Geometry check sheet. Reference: the model listing, model coordinates, mm. Face numbers are marked on the shaded views. A direction names the side the tool comes from. Coordinates: 2 decimals unless noted, no trailing zeros. Write each loop counter-clockwise with the first axis right and the second up, starting at its lowest first coordinate (ties: lowest second). Pieces come first, ordered by that corner, then holes. Notation, with made-up numbers: (-38, -5.5) -> (15, -5.5) arc R14 cw to (15, 1.5) -> close; hole circle Ø2 at (81.5, 74.25). An arc over 180 degrees is marked (long way). Put each result on its own line as item: value. Start each with the question number.
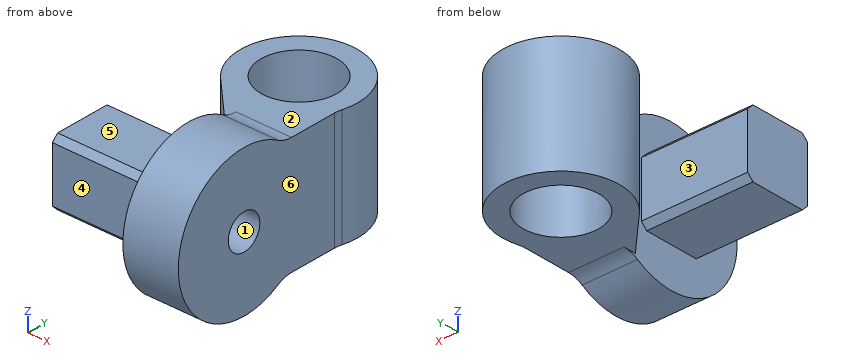
from build123d import *

# Parameters (mm, degrees)
SKETCH1_R           = 62.5
SKETCH1_R_2         = 15
BOSS_EXTRUDE1_DEPTH = 47.5
SKETCH2_R           = 32.5
BOSS_EXTRUDE2_DEPTH = 50
BOSS_EXTRUDE3_START = -47.5
BOSS_EXTRUDE3_DEPTH = 47.5
BOSS_EXTRUDE4_DEPTH = 100
FILLET1_R           = 25
SKETCH5_W           = 57
SKETCH5_H           = 57
BOSS_EXTRUDE5_DEPTH = 91
CHAMFER1_SIZE       = 5


with BuildPart() as part:
    # Sketch1 → Boss-Extrude1 (new body)
    with BuildSketch(Plane(origin=(0, 0, 0), x_dir=(0, 0, -1), z_dir=(1, 0, 0))):
        Circle(SKETCH1_R)
        Circle(SKETCH1_R_2, mode=Mode.SUBTRACT)
    extrude(amount=BOSS_EXTRUDE1_DEPTH)

    # Sketch2 → Boss-Extrude2 (add, symmetric)
    with BuildSketch(Plane.XY):
        with BuildLine():
            Line((-35.355339059, 69.644660941), (0, 34.289321881))
            Line((0, 34.289321881), (0, 55))
            ThreePointArc((0, 55), (19.134171618, 151.193976626), (-35.355339059, 69.644660941))
        make_face()
        with Locations((0, 105)):
            Circle(SKETCH2_R, mode=Mode.SUBTRACT)
    extrude(amount=BOSS_EXTRUDE2_DEPTH, both=True)

    # Sketch3 → Boss-Extrude3 (add)
    with BuildSketch(Plane(origin=(47.5, 0, 0), x_dir=(0, 0, -1), z_dir=(1, 0, 0)).offset(BOSS_EXTRUDE3_START)):
        with BuildLine():
            Line((-50, 55), (-50, 62.5))
            Line((-50, 62.5), (50, 62.5))
            Line((50, 62.5), (50, 55))
            Line((50, 55), (50, 37.5))
            ThreePointArc((50, 37.5), (40.792418173, 47.352176503), (29.685855218, 55))
            Line((29.685855218, 55), (-29.685855218, 55))
            ThreePointArc((-29.685855218, 55), (-40.792418173, 47.352176503), (-50, 37.5))
            Line((-50, 37.5), (-50, 55))
        make_face()
    extrude(amount=BOSS_EXTRUDE3_DEPTH)

    # Sketch4 → Boss-Extrude4 (add)
    with BuildSketch(Plane.XY.offset(50)):
        with BuildLine():
            Line((26.339134382, 62.5), (47.5, 62.5))
            Line((47.5, 62.5), (47.5, 89.387505004))
            ThreePointArc((47.5, 89.387505004), (39.291079432, 74.07733716), (26.339134382, 62.5))
        make_face()
    extrude(amount=-BOSS_EXTRUDE4_DEPTH)

    # Fillet1
    fillet1_edges = [part.edges().sort_by_distance(p)[0] for p in [
        (23.75, 37.5, 50),
        (23.75, 37.5, -50),
        (47.5, 89.387505004, 0),
    ]]
    fillet(fillet1_edges, radius=FILLET1_R)

    # Sketch5 → Boss-Extrude5 (add)
    with BuildSketch(Plane.ZY):
        Rectangle(SKETCH5_W, SKETCH5_H)
    extrude(amount=BOSS_EXTRUDE5_DEPTH)

    # Chamfer1
    chamfer1_edges = [part.edges().sort_by_distance(p)[0] for p in [
        (-45.5, -28.5, 28.5),
        (-45.5, 28.5, 28.5),
        (-45.5, 28.5, -28.5),
        (-45.5, -28.5, -28.5),
    ]]
    chamfer(chamfer1_edges, length=CHAMFER1_SIZE)


solid = part.part
Item 1: Go/stop test with flat-tipped pins: P1, Ø9, axis at y = -7, z = 6, coming from the +X side; P2, Ø23.5, axis at x = -38, y = -4.5, coming from the -Z side; P3, Ø6, axis at x = 35.5, z = -37, coming from the -Y side. Record where each tip stops, or that it passes through.
Item 2: Section check D-D, the plane z = 0. Enter the section's corners in (x, y), and give its area (3 significant figures).
Item 3: Mould release check, pull along Z, two halves, no side actions. Record for the marked faces 1, 2 and 3: released by +Z, released by -Z, zero draft, split by the parting line, or undercut.
Item 4: Section check C-C, the plane x = -53. Enter the section's corners in (y, z), and give its area (3 significant figures).
Item 5: Section check A-A, the plane x = 29. Enter the section's corners in (y, z).
Item 6: Access from +Z, -Z, +X, -X, +Y, -Y to the whole of each face (thin tool, end or side, straight path). Record for the marked faces 4, 5 and 6.
Item 7: Section check B-B, the plane y = 105. Enter the section's corners in (x, z).
Item 8: Scan lines: line 1 along Y through (x, z) = (0.5, -0.5); line 2 along Y through (x, z) = (26, 0); line 3 along Y through (x, z) = (-53.5, -4.5). Record each from-to range of solid material in increasing order. Write a range as [from, to].
From the geometry:
1. P1: x = 0
1. P2: z = -28.5
1. P3: y = -52.44
2. outline: (-91, -28.5) -> (0, -28.5) -> (0, -62.5) -> (47.5, -62.5) -> (47.5, -15) -> (0, -15) -> (0, 15) -> (47.5, 15) -> (47.5, 85.8) arc R25 cw to (48.33, 92.2) arc R50 ccw (long way) to (-35.36, 69.64) -> (0, 34.29) -> (0, 28.5) -> (-91, 28.5) -> close; hole circle Ø65 at (0, 105)
2. area: 14,600 mm²
3. face 1: undercut
3. face 2: released by +Z
3. face 3: zero draft
4. outline: (-28.5, -23.5) -> (-23.5, -28.5) -> (23.5, -28.5) -> (28.5, -23.5) -> (28.5, 23.5) -> (23.5, 28.5) -> (-23.5, 28.5) -> (-28.5, 23.5) -> close
4. area: 3,200 mm²
5. outline: (32.19, -53.57) arc R25 cw to (45.07, -50) -> (90.33, -50) -> (90.33, 50) -> (45.07, 50) arc R25 cw to (32.19, 53.57) arc R62.5 ccw (long way) to start; (119.67, -50) -> (145.73, -50) -> (145.73, 50) -> (119.67, 50) -> close; hole circle Ø30 at (0, 0)
6. face 4: +Z, -Z, -X, -Y
6. face 5: +Z, -X, -Y
6. face 6: +Z, -Z, +X, -Y
7. outline: (-50, -50) -> (-32.5, -50) -> (-32.5, 50) -> (-50, 50) -> close; (32.5, -50) -> (50, -50) -> (50, 50) -> (32.5, 50) -> close
8. line 1: [-62.5, -14.99], [14.99, 72.5], [137.5, 155]
8. line 2: [-62.5, -15], [15, 85.5], [124.5, 147.71]
8. line 3: [-28.5, 28.5]
